Could you check a few things on this drawing? It's one solid part, dimensions in mm from its lowest x, y, z. Give positions to 0.01 mm unless a question says otherwise; leave off trailing zeros. Order: outer loops, then holes, each group sorted by start corner. A loop starts at its lowest first (then second) coordinate and runs counter-clockwise, first axis right, second up. Notation, with made-up numbers: M 57.25,-13.5 L 81.25,-13.5 A7 cw 81.25,-5.5 Z; hole C 6,27.5 d8. An arc over 180 degrees is marked long. One line per item, written item: value. Start each with the question number.
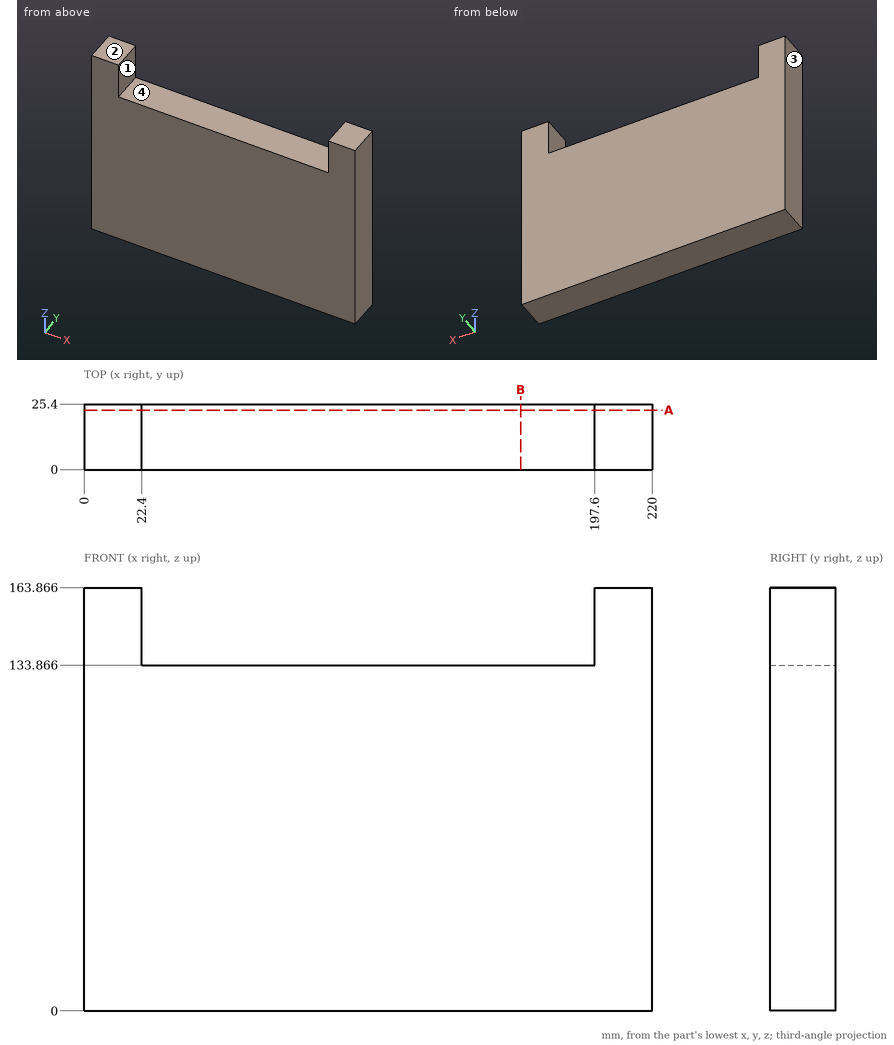
Item 1: Will this pin go through, and if not, where does the flat tip stop? P1, Ø8, axis at x = 159, y = 13, coming from the +Z side.
Item 2: I want a section at B-B on x = 169. Write out the boundary of the cut face in (y, z).
Item 3: We'd pull the mould along X, two halves only. Please class the marked faces 1, 2, 3 and 4: +X half, -X half, draft (parallel to the pull), parting line (faces both ways), or undercut.
Item 4: Please list where these lines run through material, in increasing order: probe 1 along X at (y, z) = (1.5, 147.5); probe 2 along Z at (x, y) = (121, 6). Write a range as [from, to].
Item 5: I want a section at A-A on y = 23. Write out the boundary of the cut face in (x, z).
Answer below:
1. P1: stops at z = 133.87
2. outline: M 0,0 L 25.4,0 L 25.4,133.87 L 0,133.87 Z
3. face 1: undercut
3. face 2: draft
3. face 3: -X half
3. face 4: undercut
4. probe 1: x = [0, 22.4], [197.6, 220]
4. probe 2: z = [0, 133.87]
5. outline: M 0,0 L 220,0 L 220,163.87 L 197.6,163.87 L 197.6,133.87 L 22.4,133.87 L 22.4,163.87 L 0,163.87 Z
